from build123d import *

# Parameters (mm, degrees)
CUT_EXTRUDE1_DEPTH  = 5
CUT_EXTRUDE12_DEPTH = 5.5
CHAMFER1_SIZE       = 2


with BuildPart() as part:
    # Sketch1 → Revolve1 (revolve)
    with BuildSketch(Plane(origin=(0, 0, 0), x_dir=(1, 0, 0), z_dir=(0, 1, 0))):
        Polygon((0, 0), (0, -400), (20, -400), (20, -269.514398681), (22.5, -269.514398681), (22.5, -220), (31.046216184, -220), (31.046216184, -140), (18.413082613, -140), (18.413082613, -130), (31.046216184, -130), (31.046216184, -30), (22.5, -30), (22.5, 0), align=None)
    revolve(axis=Axis((0, 0, 0), (0, 0, 1)))

    # Sketch3 → Cut-Extrude1 (cut)
    with BuildSketch(Plane(origin=(0, 20, 400), x_dir=(0, 0, 1), z_dir=(0, -1, 0))):
        with BuildLine():
            Line((-25, 6), (-75, 6))
            ThreePointArc((-75, 6), (-81, 0), (-75, -6))
            Line((-75, -6), (-25, -6))
            ThreePointArc((-25, -6), (-19, 0), (-25, 6))
        make_face()
    extrude(amount=CUT_EXTRUDE1_DEPTH, mode=Mode.SUBTRACT)

    # Sketch32 → Cut-Extrude12 (cut)
    with BuildSketch(Plane(origin=(0, 31.046216184, 220), x_dir=(0, 0, 1), z_dir=(0, -1, 0))):
        with BuildLine():
            Line((-27, 7), (-67, 7))
            ThreePointArc((-67, 7), (-74, 0), (-67, -7))
            Line((-67, -7), (-27, -7))
            ThreePointArc((-27, -7), (-20, 0), (-27, 7))
        make_face()
    extrude(amount=CUT_EXTRUDE12_DEPTH, mode=Mode.SUBTRACT)

    # Chamfer1
    chamfer1_edges = [part.edges().sort_by_distance(p)[0] for p in [
        (-20, 0, 400),
    ]]
    chamfer(chamfer1_edges, length=CHAMFER1_SIZE)


solid = part.part
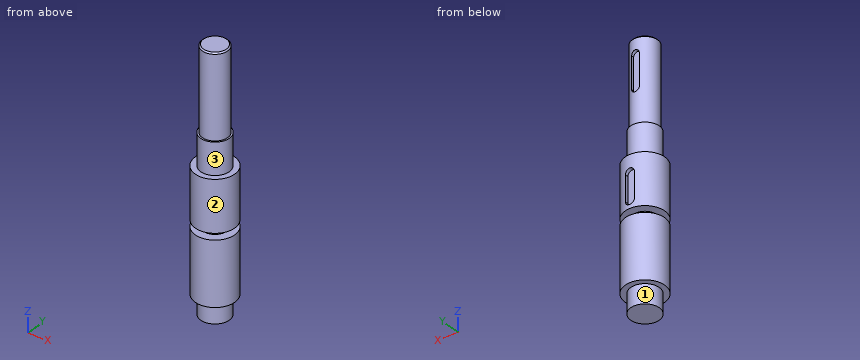
Check sheet for the modelled part. Datum: model origin and axes. Units: mm. Face numbers are marked on the shaded views. A direction names the side the tool comes from. Round coordinates to 2 decimals unless told otherwise and drop trailing zeros. Write each loop counter-clockwise with the first axis right and the second up, starting at its lowest first coordinate (ties: lowest second). Pieces come first, ordered by that corner, then holes. Notation, with made-up numbers: (-39.5, 45.5) - (-21.5, 45.5) arc R22 ccw to (-21.5, 57.5) - close; hole circle Ø8 at (-37.5, -12). An arc over 180 degrees is marked (long way). Return JSON: item names as keys, results as strings.
Q1. Depth check by flat-ended pin: P1, Ø13, axis at x = 0.5, z = 353, coming from the +Y side; P2, Ø12, axis at y = 3, z = 274.5, coming from the +X side; P3, Ø8, axis at y = 8, z = 275, coming from the -X side; P4, Ø3, axis at x = -18, y = -5, coming from the -Z side. Enter the tip coordinate at first touch or a pass-through.
Returned:
{"P1": "stops at y = 19.08", "P2": "stops at x = 22.5", "P3": "stops at x = -19.6", "P4": "stops at z = 0"}
Q2. Cross-section at C-C (z = 68). Record the boundary of the cut face in (x, y), then the cut area to 3 significant figures.
Returned:
{"outline": "circle Ø62.09 at (0, 0)", "area": "3,030 mm²"}
Q3. Cross-section at B-B (z = 187). Record the boundary of the cut face in (x, y).
Returned:
{"outline": "(-7, 25.55) - (-7, 30.25) arc R31.05 ccw (long way) to (7, 30.25) - (7, 25.55) - close"}
Q4. Cross-section at A-A (z = 291.5). Record the boundary of the cut face in (x, y).
Returned:
{"outline": "circle Ø40 at (0, 0)"}
Q5. Access from +Z, -Z, +X, -X, +Y, -Y to the whole of each face (thin tool, end or side, straight path). Record for the marked faces 1, 2 and 3.
Returned:
{"face 1": "-Z", "face 2": "+Z, -Z", "face 3": "+Z"}
Q6. Scan lines: L1, parallel to Z at x = -24, y = 14; L2, parallel to Z at x = -21.5, y = -2; L3, parallel to Y at x = -13.5, z = 253. Record each from-to range of solid material in increasing order. Write a range as from..to.
Returned:
{"L1": "z = 30..130, 140..220", "L2": "z = 0..130, 140..269.51", "L3": "y = -18..18"}
